For this review, take the finished solid that the model builds, in its own axes (mm). Give positions to 0.01 mm unless a question says otherwise; leave off trailing zeros. Write each loop counter-clockwise with the first axis right and the second up, starting at its lowest first coordinate (ties: lowest second). Pieces come first, ordered by that corner, then holes. Notation, with made-up numbers: (41, -36) -> (70, -36) arc R13 cw to (70, -17) -> close; hole circle Ø9 at (38, 13). An arc over 180 degrees is marked (long way). Answer as CSV lines item,"result".
```python
from build123d import *

# Parameters (mm, degrees)
SKETCH1_W          = 253
SKETCH1_H          = 126
BASE_FLANGE1_DEPTH = 1


# Sheet-metal steps are written as plain solids
with BuildPart() as part:
    # Sketch1 → Base-Flange1 (new body)
    with BuildSketch(Plane.XY):
        Rectangle(SKETCH1_W, SKETCH1_H)
        with BuildLine():
            Line((-81, -7.2), (-74.538477631, -7.2))
            ThreePointArc((-74.538477631, -7.2), (-73.773110766, -7.047759065), (-73.124264069, -6.614213562))
            Line((-73.124264069, -6.614213562), (-70.005025253, -3.494974747))
            Line((-70.005025253, -3.494974747), (-66.885786438, -0.375735931))
            ThreePointArc((-66.885786438, -0.375735931), (-66.452240935, 0.273110766), (-66.3, 1.038477631))
            Line((-66.3, 1.038477631), (-66.3, 39.2))
            ThreePointArc((-66.3, 39.2), (-66.885786438, 40.614213562), (-68.3, 41.2))
            Line((-68.3, 41.2), (-93.7, 41.2))
            ThreePointArc((-93.7, 41.2), (-95.114213562, 40.614213562), (-95.7, 39.2))
            Line((-95.7, 39.2), (-95.7, 19.75))
            Line((-95.7, 19.75), (-95.7, 1.038477631))
            ThreePointArc((-95.7, 1.038477631), (-95.547759065, 0.273110766), (-95.114213562, -0.375735931))
            Line((-95.114213562, -0.375735931), (-94.064941978, -1.425007515))
            Line((-94.064941978, -1.425007515), (-91.994974747, -3.494974747))
            Line((-91.994974747, -3.494974747), (-88.875735931, -6.614213562))
            ThreePointArc((-88.875735931, -6.614213562), (-88.226889234, -7.047759065), (-87.461522369, -7.2))
            Line((-87.461522369, -7.2), (-81, -7.2))
        make_face(mode=Mode.SUBTRACT)
    extrude(amount=-BASE_FLANGE1_DEPTH)


solid = part.part
```
Q1. Add section B-B (x = -78.5). Write out the cut boundary in (y, z).
Answer block:
outline,"(-63, -1) -> (-7.2, -1) -> (-7.2, 0) -> (-63, 0) -> close; (41.2, -1) -> (63, -1) -> (63, 0) -> (41.2, 0) -> close"
Q2. Add section C-C (z = -0.65). Write out the cut boundary in (x, y) (3 decimals), plus the area to 3 significant figures.
Answer block:
outline,"(-126.5, -63) -> (126.5, -63) -> (126.5, 63) -> (-126.5, 63) -> close; hole (-95.7, 1.038) arc R2 ccw to (-95.114, -0.376) -> (-88.876, -6.614) arc R2 ccw to (-87.462, -7.2) -> (-74.538, -7.2) arc R2 ccw to (-73.124, -6.614) -> (-66.886, -0.376) arc R2 ccw to (-66.3, 1.038) -> (-66.3, 39.2) arc R2 ccw to (-68.3, 41.2) -> (-93.7, 41.2) arc R2 ccw to (-95.7, 39.2) -> close"
area,"30,500 mm2"
Q3. To check wall thickness, follow probe 1 along Y at (x, z) = (-75, -0.6); probe 2 along X at (y, z) = (38, -0.2). State the ranges of each line that lie inside material, in increasing order. Write a range as [from, to].
Answer block:
probe 1,"y = [-63, -7.2], [41.2, 63]"
probe 2,"x = [-126.5, -95.7], [-66.3, 126.5]"
Q4. Add section A-A (y = 20). Write out the cut boundary in (x, z), plus the area to 3 significant figures.
Answer block:
outline,"(-126.5, -1) -> (-95.7, -1) -> (-95.7, 0) -> (-126.5, 0) -> close; (-66.3, -1) -> (126.5, -1) -> (126.5, 0) -> (-66.3, 0) -> close"
area,"224 mm2"
